Autodesk Inventor part; units mm, degrees
ref_plane "YZ Plane" through (0, 0, 0) normal (1, 0, 0) x (0, 1, 0)
ref_plane "XZ Plane" through (0, 0, 0) normal (0, 1, 0) x (-1, 0, 0)
ref_plane "XY Plane" through (0, 0, 0) normal (0, 0, 1) x (1, 0, 0)
sketch "Sketch1" plane through (0, 0, 0) normal (0, 0, 1) x (1, 0, 0)
  line L0 (0, 0) -> (44.45, 0)
  line L1 (44.45, 0) -> (44.45, -50.8)
  line L2 (44.45, -50.8) -> (0, -50.8)
  line L3 (0, -50.8) -> (0, 0)
  line L4 (6.35, 0) -> (12.7, 0)
  line L5 (12.7, 0) -> (12.7, 12.7)
  line L6 (12.7, 12.7) -> (6.35, 12.7)
  line L7 (6.35, 12.7) -> (6.35, 0)
  line L8 (31.75, 0) -> (38.1, 0)
  line L9 (38.1, 0) -> (38.1, 12.7)
  line L10 (38.1, 12.7) -> (31.75, 12.7)
  line L11 (31.75, 12.7) -> (31.75, 0)
  circle A0 centre (22.225, -25.4) radius 9.5885
  dimension "d0" = 44.45
  dimension "d1" = 50.8
  dimension "d3" = 6.35
  dimension "d4" = 6.35
  dimension "d5" = 6.35
  dimension "d6" = 19.05
  dimension "d9" = 19.177
  dimension "d20" = 12.7
  dimension "d21" = 22.225
  dimension "d22" = 25.4
  dimension "d25" = 6.35
extrude "Extrusion1" add sketch "Sketch1" against normal blind 12.7 contours L0 L1 L2 L3 | L7 L6 L5 L0 | L11 L10 L9 L0 | A0
sketch "Sketch2" plane through (0, 0, 0) normal (0, 0, 1) x (1, 0, 0)
  circle A0 centre (22.225, -25.4) radius 8.8265
  line L0 (0, -50.8) -> (0, 0)
  dimension "d10" = 17.653
  dimension "d23" = 22.225
extrude "Extrusion2" cut sketch "Sketch2" against normal blind 12.7
sketch "Sketch3" plane through (38.1, 0, 0) normal (1, 0, 0) x (0, 0, -1)
  line L0 (12.7, 12.7) -> (12.7, 0)
  line L1 (0, 12.7) -> (12.7, 12.7)
  circle A0 centre (6.35, 6.35) radius 2.4447
  dimension "d13" = 4.8895
  dimension "d14" = 6.35
  dimension "d15" = 6.35
extrude "Extrusion3" cut sketch "Sketch3" against normal through all
fillet "Fillet2" radius 6.35 2 edges at (44.45, -50.8, -6.35) (0, -50.8, -6.35)
fillet "Fillet3" radius 3.175 6 edges at (38.1, 0, -6.35) (12.7, 0, -6.35) (31.75, 0, -6.35) (6.35, 0, -6.35) (44.45, 0, -6.35) (0, 0, -6.35)
properties part number "Needle Bearing Mount v2"
Verification items for the finished model (mm, model axes). A direction names the side the tool comes from. Coordinates: 2 decimals unless noted, no trailing zeros. Loops run counter-clockwise (first coordinate to the right, second up) from the corner with the lowest first, then second, coordinate; pieces in that order, holes last. Notation, with made-up numbers: (41, 20.25) -> (99, 20.25) arc R15 cw to (99, 45.25) -> close; hole circle Ø7 at (-34.5, 55). An arc over 180 degrees is marked (long way). Answer in a Markdown table with one row per item. Add a question column.
1. Material ranges on probe 1 along Y at (x, z) = (37, -6.25); probe 2 along Y at (x, z) = (26, -10.25); probe 3 along X at (y, z) = (-26, -1.75), recorded low to high. Write a range as [from, to].
2. Depth check by flat-ended pin: P1, Ø3, axis at y = 10, z = -7.5, coming from the +X side; P2, Ø4, axis at y = 6.35, z = -6.35, coming from the +X side; P3, Ø3, axis at y = 7.5, z = -7.5, coming from the -X side. Enter the tip coordinate at first touch or a pass-through.
3. Access from +Z, -Z, +X, -X, +Y, -Y to the whole of each face (thin tool, end or side, straight path). Record for faces 4 (the face through (0, -24, -6)), 5 (the face through (12.7, 9, -6)), 6 (the face through (6.35, 9, -6)).
4. Draft check along X on faces 1 (the face through (5.44, 0.95, -6.44)), 2 (the face through (22, 0, -6)), 3 (the face through (38.1, 9, -6)). Enter one of: +X half, -X half, draft (parallel to the pull), parting line (faces both ways), or undercut.
5. Section check A-A, the plane z = -6.35. Give the number of separate pieces and of enclosed holes in the cut face, then the cut area to 3 significant figures.
6. Section check D-D, the plane x = 30. Enter the section's corners in (y, z).
7. Section check B-B, the plane y = 6.35. Enter the section's corners in (x, z).
Derived:
| question | item | result |
|---|---|---|
| 1 | probe 1 | y = [-50.8, 3.91], [8.79, 12.7] |
| 1 | probe 2 | y = [-50.8, -33.38], [-17.42, 0] |
| 1 | probe 3 | x = [0, 13.42], [31.03, 44.45] |
| 2 | P1 | stops at x = 38.1 |
| 2 | P2 | passes through |
| 2 | P3 | stops at x = 6.35 |
| 3 | face 4 | +Z, -Z, -X, +Y, -Y |
| 3 | face 5 | +Z, -Z, +Y |
| 3 | face 6 | +Z, -Z, -X, +Y |
| 4 | face 1 | -X half |
| 4 | face 2 | undercut |
| 4 | face 3 | +X half |
| 5 | separate pieces | 3 |
| 5 | enclosed holes | 1 |
| 5 | area | 2,100 mm² |
| 6 | outline | (-50.8, -12.7) -> (-29.58, -12.7) -> (-29.58, 0) -> (-50.8, 0) -> close; (-21.22, -12.7) -> (0.34, -12.7) -> (0.34, 0) -> (-21.22, 0) -> close |
| 7 | outline | (6.35, -12.7) -> (12.7, -12.7) -> (12.7, -8.79) -> (6.35, -8.79) -> close; (6.35, -3.91) -> (12.7, -3.91) -> (12.7, 0) -> (6.35, 0) -> close; (31.75, -12.7) -> (38.1, -12.7) -> (38.1, -8.79) -> (31.75, -8.79) -> close; (31.75, -3.91) -> (38.1, -3.91) -> (38.1, 0) -> (31.75, 0) -> close |
